```python
from build123d import *

# Parameters (mm, degrees)
PAD_DEPTH    = 20.32
POCKET_DEPTH = 21


with BuildPart() as part:
    # Sketch → Pad (new body)
    with BuildSketch(Plane.XY):
        Polygon((0, 0), (0, 2.51), (5, 2.51), (4.999966, 8.51), (123.5, 8.51), (123.5, 2.51), (128.5, 2.51), (128.5, 0), align=None)
    extrude(amount=PAD_DEPTH)

    # Sketch002 → Pocket (cut)
    with BuildSketch(Plane.XZ):
        with BuildLine():
            ThreePointArc((20, 15.000243), (16.464298, 13.535707), (14.999762, 10.000005))
            Line((14.999762, 10.000005), (14.999762, -25.27))
            Line((14.999762, -25.27), (45, -25.27))
            Line((45, -25.27), (45, 10.000238))
            ThreePointArc((45, 10.000238), (43.518366, 13.552956), (39.951518, 15.000243))
            Line((39.951518, 15.000243), (20, 15.000243))
        make_face()
    extrude(amount=-POCKET_DEPTH, mode=Mode.SUBTRACT)


solid = part.part
```
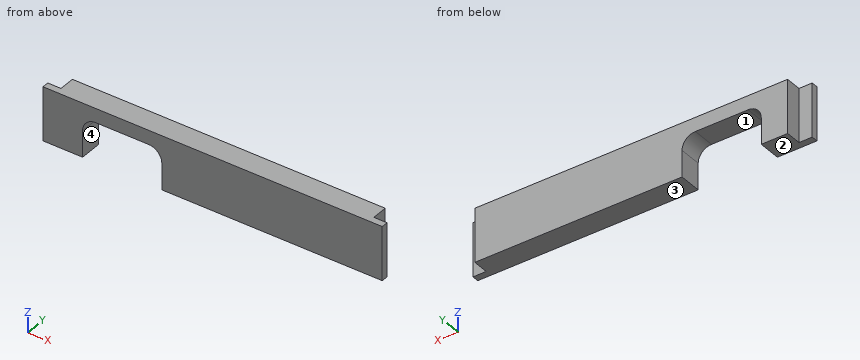
Part model, mm, in its own coordinate system. Face numbers are marked on the shaded views. A direction names the side the tool comes from. Round coordinates to 2 decimals unless told otherwise and drop trailing zeros. Write each loop counter-clockwise with the first axis right and the second up, starting at its lowest first coordinate (ties: lowest second). Pieces come first, ordered by that corner, then holes.
Item 1: Cut at C-C, the plane z = 4. Give the cut face in (x, y), plus the area to 3 significant figures.
Results:
outline: (0, 0) - (15, 0) - (15, 8.51) - (5, 8.51) - (5, 2.51) - (0, 2.51) - close; (45, 0) - (128.5, 0) - (128.5, 2.51) - (123.5, 2.51) - (123.5, 8.51) - (45, 8.51) - close
area: 778 mm2
Item 2: Two-plate mould, pull along X, no slides. Class the marked faces 3 and 4: +X half, -X half, draft (parallel to the pull), parting line (faces both ways), or undercut.
Results:
face 3: draft
face 4: undercut
Item 3: Which spindle directions (+Z, -Z, +X, -X, +Y, -Y) get a long thin tool onto all of the face, cutting with end or side? Do the marked faces 1 and 2. Say none if no direction does.
Results:
face 1: -Z, +Y, -Y
face 2: -Z, +X, -X, +Y, -Y
Item 4: Cut at D-D, the plane x = 32.5. Give the cut face in (y, z).
Results:
outline: (0, 15) - (8.51, 15) - (8.51, 20.32) - (0, 20.32) - close
Item 5: Drop flat-ended pins along their axis: pin 1 Ø4.5 at (y, z) = (3, 6) entering from -X; pin 2 Ø5.5 at (x, z) = (2, 12) entering from +Y; pin 3 Ø4.5 at (x, y) = (28.5, 6) entering from -Z. Give the stop position or say it passes through.
Results:
pin 1: stops at x = 0
pin 2: stops at y = 2.51
pin 3: stops at z = 15
Item 6: Probe L1, parallel to X at y = 7, z = 10.25; L2, parallel to X at y = 1, z = 9.5; L3, parallel to X at y = 4.5, z = 17.25. List the from-to ranges inside material, lowest first.
Results:
L1: x = 5 to 15.01, 44.99 to 123.5
L2: x = 0 to 15, 45 to 128.5
L3: x = 5 to 123.5
Item 7: Cut at A-A, the plane z = 12.25. Give the cut face in (x, y), plus the area to 3 significant figures.
Results:
outline: (0, 0) - (15.53, 0) - (15.53, 8.51) - (5, 8.51) - (5, 2.51) - (0, 2.51) - close; (44.47, 0) - (128.5, 0) - (128.5, 2.51) - (123.5, 2.51) - (123.5, 8.51) - (44.47, 8.51) - close
area: 787 mm2
Item 8: Cut at B-B, the plane y = 6. Give the cut face in (x, z), plus the area to 3 significant figures.
Results:
outline: (5, 0) - (15, 0) - (15, 10) arc R5 cw to (20, 15) - (39.95, 15) arc R5 cw to (45, 10) - (45, 0) - (123.5, 0) - (123.5, 20.32) - (5, 20.32) - close
area: 1,970 mm2
